from build123d import *

# Parameters (mm, degrees)
ESQUISSE1_W             = 80
ESQUISSE1_H             = 27.5
BOSS_EXTRU_1_DEPTH      = 4
ESQUISSE2_R             = 2
ESQUISSE2_W             = 40
ESQUISSE2_H             = 20
ENL_V_MAT_EXTRU_1_DEPTH = 43.486027115
ENL_V_MAT_EXTRU_2_DEPTH = 43.486027115
CONG_1_R                = 5


with BuildPart() as part:
    # Esquisse1 → Boss.-Extru.1 (new body)
    with BuildSketch(Plane.XY):
        Rectangle(ESQUISSE1_W, ESQUISSE1_H)
    extrude(amount=BOSS_EXTRU_1_DEPTH)

    # Esquisse2 → Enlèv. mat.-Extru.1 (cut, through all)
    with BuildSketch(Plane(origin=(0, 0, 0), x_dir=(-1, 0, 0), z_dir=(0, 0, -1))):
        with Locations((-23.9, 1.35)):
            Circle(ESQUISSE2_R)
        with Locations(Location((-23.9, -8.85, 0), (0, 0, 180))):
            Circle(ESQUISSE2_R)
        with Locations((23.9, -8.85)):
            Circle(ESQUISSE2_R)
        with Locations(Location((23.9, 1.35, 0), (0, 0, 180))):
            Circle(ESQUISSE2_R)
        with Locations((0, -3.75)):
            Rectangle(ESQUISSE2_W, ESQUISSE2_H)
    extrude(amount=-ENL_V_MAT_EXTRU_1_DEPTH, mode=Mode.SUBTRACT)

    # Esquisse3 → Enlèv. mat.-Extru.2 (cut, through all)
    with BuildSketch(Plane(origin=(0, 0, 0), x_dir=(-1, 0, 0), z_dir=(0, 0, -1))):
        Polygon((31.15, -13.75), (35.35, -13.75), (35.35, -6.95), (36.75, -6.95), (36.75, -3.75), (35.35, -3.75), (35.35, 3.25), (31.15, 3.25), (31.15, -3.75), (29.75, -3.75), (29.75, -6.95), (31.15, -6.95), align=None)
        Polygon((-31.15, -13.75), (-31.15, -6.95), (-29.75, -6.95), (-29.75, -3.75), (-31.15, -3.75), (-31.15, 3.25), (-35.35, 3.25), (-35.35, -3.75), (-36.75, -3.75), (-36.75, -6.95), (-35.35, -6.95), (-35.35, -13.75), align=None)
    extrude(amount=-ENL_V_MAT_EXTRU_2_DEPTH, mode=Mode.SUBTRACT)

    # Congé1
    cong_1_edges = [part.edges().sort_by_distance(p)[0] for p in [
        (-40, 13.75, 2),
        (40, 13.75, 2),
    ]]
    fillet(cong_1_edges, radius=CONG_1_R)


solid = part.part
Can you work these out from the model? Positions are in its coordinate system, mm. A direction names the side the tool comes from. Coordinates: 2 decimals unless noted, no trailing zeros. Write each loop counter-clockwise with the first axis right and the second up, starting at its lowest first coordinate (ties: lowest second). Pieces come first, ordered by that corner, then holes. Notation, with made-up numbers: (52, 22) -> (69, 22) arc R20 ccw to (69, 53) -> close; hole circle Ø11 at (82, -39.75). An arc over 180 degrees is marked (long way). Write each question's results on one line, items separated by ' | '. Start each with the question number.
Q1. Imagine slicing it at C-C (y = 1.35). Write out the boundary of the cut face in (x, z).
Q2. Imagine slicing it at B-B (y = -2.25). Write out the boundary of the cut face in (x, z), then the cut area to 3 significant figures.
Q3. Imagine slicing it at A-A (x = -23.9). Write out the boundary of the cut face in (y, z).
Q4. Imagine slicing it at D-D (z = 3.3). State how many separate pieces and enclosed holes the cut face has, then the cut area to 3 significant figures.
Q5. I'm going to push flat-ended pins straight in: pin 1 (1.2 mm diameter, centred on x = 8, z = 2.5, fed in from -Y); pin 2 (3.5 mm diameter, centred on x = 23.9, y = 1.35, fed in from +Z); pin 3 (1.5 mm diameter, centred on x = 25.5, y = -6.5, fed in from -Z). Where does each tip first touch, or does it pass through?
Q6. We'd pull the mould along X, two halves only. Please class faces 1 (the face through (0, 13.75, 2)), 2 (the face through (-38.57, 12.25, 2.03)), 3 (the face through (-35.35, 0, 2)): +X half, -X half, draft (parallel to the pull), parting line (faces both ways), or undercut.
Q7. On a 3-axis mill with a long thin cutter (end or side, diameter ignored), from which of +Z, -Z, +X, -X, +Y, -Y can I reach the whole of each face in a straight line? I mean faces 4 (the face through (-40, -3, 2)), 5 (the face through (31.15, 0, 2)), 6 (the face through (-36, -3.75, 2)). Say none if no direction works.
Q8. If I drill on probe 1 along X at (y, z) = (-8.75, 0.7); probe 2 along X at (y, z) = (-1, 2.2); probe 3 along Y at (x, z) = (23.9, 1.7), over which ranges is the centre line in solid material (lowest first)?
Taken from the geometry:
1) outline: (-40, 0) -> (-35.35, 0) -> (-35.35, 4) -> (-40, 4) -> close; (-31.15, 0) -> (-25.9, 0) -> (-25.9, 4) -> (-31.15, 4) -> close; (-21.9, 0) -> (-20, 0) -> (-20, 4) -> (-21.9, 4) -> close; (20, 0) -> (21.9, 0) -> (21.9, 4) -> (20, 4) -> close; (25.9, 0) -> (31.15, 0) -> (31.15, 4) -> (25.9, 4) -> close; (35.35, 0) -> (40, 0) -> (40, 4) -> (35.35, 4) -> close
2) outline: (-40, 0) -> (-35.35, 0) -> (-35.35, 4) -> (-40, 4) -> close; (-31.15, 0) -> (-20, 0) -> (-20, 4) -> (-31.15, 4) -> close; (20, 0) -> (31.15, 0) -> (31.15, 4) -> (20, 4) -> close; (35.35, 0) -> (40, 0) -> (40, 4) -> (35.35, 4) -> close | area: 126 mm^2
3) outline: (-13.75, 0) -> (-10.85, 0) -> (-10.85, 4) -> (-13.75, 4) -> close; (-6.85, 0) -> (-0.65, 0) -> (-0.65, 4) -> (-6.85, 4) -> close; (3.35, 0) -> (13.75, 0) -> (13.75, 4) -> (3.35, 4) -> close
4) separate pieces: 1 | enclosed holes: 4 | area: 1,180 mm^2
5) pin 1: stops at y = 6.25 | pin 2: passes through | pin 3: stops at z = 0
6) face 1: draft | face 2: -X half | face 3: undercut
7) face 4: +Z, -Z, -X, +Y, -Y | face 5: +Z, -Z, -Y | face 6: +Z, -Z
8) probe 1: x = -40 to -35.35, -31.15 to -25.9, -21.9 to -20, 20 to 21.9, 25.9 to 31.15, 35.35 to 40 | probe 2: x = -40 to -35.35, -31.15 to -20, 20 to 31.15, 35.35 to 40 | probe 3: y = -13.75 to -10.85, -6.85 to -0.65, 3.35 to 13.75
